from build123d import *

# Parameters (mm, degrees)
F0_W        = 6.5
F0_H        = 20
F1_DEPTH    = 22.35
F3_DEPTH    = 25
F4_T1_DEPTH = 27.35


# Not quite as in the source:
# - a fillet or chamfer that OpenCascade refuses, or shapes differently, is made with other operations: its cross-section is extruded or revolved along the edge and cut away or added


with BuildPart() as f1:
    # F0 (on Top) → F1 (new body)
    with BuildSketch(Plane.XY):
        with Locations((3.25, 10)):
            Rectangle(F0_W, F0_H)
    extrude(amount=F1_DEPTH)

    # F2 (on face) → F3 (cut)
    with BuildSketch(Plane.XZ):
        with BuildLine():
            ThreePointArc((6.5, 22.35), (3.25, 25.6), (0, 22.35))
            Line((0, 22.35), (6.5, 22.35))
        make_face()
        with BuildLine():
            Line((6.5, 22.35), (0, 22.35))
            ThreePointArc((0, 22.35), (3.25, 19.1), (6.5, 22.35))
        make_face()
    extrude(amount=-F3_DEPTH, mode=Mode.SUBTRACT)

    # F4: fillet of radius 1 on 4 edges, made by hand

    # F4_s2 → F4_t1 (cut)
    with BuildSketch(Plane.XY.offset(-2.5)):
        with BuildLine():
            ThreePointArc((5.5, 0), (6.2071067812, 0.2928932188), (6.5, 1))
            Line((6.5, 1), (6.5, 0))
            Line((6.5, 0), (5.5, 0))
        make_face()
        with BuildLine():
            ThreePointArc((0, 1), (0.2928932188, 0.2928932188), (1, 0))
            Line((1, 0), (0, 0))
            Line((0, 0), (0, 1))
        make_face()
        with BuildLine():
            ThreePointArc((5.5, 20), (6.2071067812, 19.7071067812), (6.5, 19))
            Line((6.5, 19), (6.5, 20))
            Line((6.5, 20), (5.5, 20))
        make_face()
        with BuildLine():
            ThreePointArc((0, 19), (0.2928932188, 19.7071067812), (1, 20))
            Line((1, 20), (0, 20))
            Line((0, 20), (0, 19))
        make_face()
    extrude(amount=F4_T1_DEPTH, mode=Mode.SUBTRACT)


solid = f1.part
CAD build for the part. Positions are in the model's coordinates, mm. Round coordinates to 2 decimals unless told otherwise and drop trailing zeros. Write each loop counter-clockwise with the first axis right and the second up, starting at its lowest first coordinate (ties: lowest second). Pieces come first, ordered by that corner, then holes. Notation, with made-up numbers: M 20.5,21.5 L 31.5,21.5 A15 cw 31.5,42.5 Z; hole C 89,38 d8. An arc over 180 degrees is marked long. Put each result on its own line as item: value. Start each with the question number.
1) Pin check, flat tip, straight feed: pin 1 Ø2 at (x, y) = (4.5, 4) entering from +Z. Stop position of the tip, or through.
2) Drill centre lines: probe 1 along Z at (x, y) = (1, 6.25); probe 2 along Z at (x, y) = (2.5, 9.75); probe 3 along Y at (x, z) = (0.75, 19). Where is each one in solid material? Low to high. Write a range as [from, to].
3) Saw through at A-A, the plane x = 2. Write the cut outline in (y, z), and give its area (3 significant figures).
4) Saw through at B-B, the plane y = 14.25. Write the cut outline in (x, z).
Resolved:
1. pin 1: z = 20
2. probe 1: [0, 20]
2. probe 2: [0, 19.19]
2. probe 3: [0.03, 19.97]
3. outline: M 0,0 L 20,0 L 20,19.35 L 0,19.35 Z
3. area: 387 mm²
4. outline: M 0,0 L 6.5,0 L 6.5,22.35 A3.25 cw 0,22.35 Z
